```python
from build123d import *

# Parameters (mm, degrees)
SKETCH_1_R      = 5.05
SKETCH_1_R_2    = 2.05
SKETCH_1_R_3    = 3.701732688
EXTRUDE_1_DEPTH = 2


with BuildPart() as part:
    # 草图1 → 凸台-拉伸1 (new body)
    with BuildSketch(Plane.XY):
        with BuildLine():
            Line((-80.687991051, 42.414942906), (-80.687991051, -192.585057094))
            ThreePointArc((-80.687991051, -192.585057094), (-52.757273194, -260.015774951), (-120.187991051, -232.085057094))
            Line((-120.187991051, -232.085057094), (-140.687991051, -211.585057094))
            Line((-140.687991051, -211.585057094), (-140.687991051, 61.414942906))
            Line((-140.687991051, 61.414942906), (-120.187991051, 81.914942906))
            ThreePointArc((-120.187991051, 81.914942906), (-52.757273194, 109.845660763), (-80.687991051, 42.414942906))
        make_face()
        with Locations((-80.687991051, 81.914942906)):
            Circle(SKETCH_1_R, mode=Mode.SUBTRACT)
        with Locations((-80.687991051, 56.914942906)):
            Circle(SKETCH_1_R_2, mode=Mode.SUBTRACT)
        with Locations((-108.618708908, 53.984225049)):
            Circle(SKETCH_1_R_3, mode=Mode.SUBTRACT)
        with Locations((-55.687991051, 81.914942906)):
            Circle(SKETCH_1_R_2, mode=Mode.SUBTRACT)
        with Locations((-105.687991051, 81.914942906)):
            Circle(SKETCH_1_R_2, mode=Mode.SUBTRACT)
        with Locations((-80.687991051, 106.914942906)):
            Circle(SKETCH_1_R_2, mode=Mode.SUBTRACT)
        with Locations(Location((-80.687991051, -257.085057094, 0), (0, 0, 180))):
            Circle(SKETCH_1_R_2, mode=Mode.SUBTRACT)
        with Locations(Location((-105.687991051, -232.085057094, 0), (0, 0, 180))):
            Circle(SKETCH_1_R_2, mode=Mode.SUBTRACT)
        with Locations(Location((-55.687991051, -232.085057094, 0), (0, 0, 180))):
            Circle(SKETCH_1_R_2, mode=Mode.SUBTRACT)
        with Locations(Location((-108.618708908, -204.154339237, 0), (0, 0, 180))):
            Circle(SKETCH_1_R_3, mode=Mode.SUBTRACT)
        with Locations(Location((-80.687991051, -207.085057094, 0), (0, 0, 180))):
            Circle(SKETCH_1_R_2, mode=Mode.SUBTRACT)
        with Locations(Location((-80.687991051, -232.085057094, 0), (0, 0, 180))):
            Circle(SKETCH_1_R, mode=Mode.SUBTRACT)
    extrude(amount=EXTRUDE_1_DEPTH)


solid = part.part
```
Geometry: final body of the model. Coordinates: model frame, mm. Coordinates: 2 decimals unless noted, no trailing zeros. Order: outer loops, then holes, each group sorted by start corner. A loop starts at its lowest first (then second) coordinate and runs counter-clockwise, first axis right, second up. Notation, with made-up numbers: M 62,87 L 81,87 A27 ccw 81,103 Z; hole C 55.5,87 d11. An arc over 180 degrees is marked long. Answer in a Markdown table with one row per item. Add a question column.
Q1. Contact query for flat-ended pins moving along their axis: P1, Ø6.5, axis at x = -55.69, y = -232.09, coming from the +Z side; P2, Ø2.5, axis at x = -105.69, y = -232.09, coming from the +Z side; P3, Ø1, axis at y = -145.5, z = 0.5, coming from the +X side. Output: stop coordinate, or through.
Q2. Section query C-C on x = -98.5. Return the cut outline in (y, z).
Q3. Line query: L1, parallel to Y at x = -48.5, z = 0.6; L2, parallel to X at y = -21.5, z = 1.8; L3, parallel to Y at x = -55.5, z = 1.25. Output: solid intervals per line, ascending.
Q4. Section query B-B on y = -22. Return the cut outline in (x, z).
Q5. Section query A-A on z = 0.8. Count the separate pieces of the cut face and the enclosed holes in it, and give its area (3 significant figures).
Q6. Mould query, pull axis X, two halves, no side actions, for faces 1 (the flat face through (-130.294, -221.979, 0.986)), 2 (the cylindrical face through (-76.023, 79.981, 0.986)), 3 (the cylindrical face through (-53.69, 110.75, 0.99)). Classes: released by +X, released by -X, zero draft, split by the parting line, or undercut.
Completed:
| question | item | result |
|---|---|---|
| 1 | P1 | stops at z = 2 |
| 1 | P2 | passes through |
| 1 | P3 | stops at x = -80.69 |
| 2 | outline | M -267.34,0 L 117.17,0 L 117.17,2 L -267.34,2 Z |
| 3 | L1 | y = -254.98 to -209.19, 59.02 to 104.81 |
| 3 | L2 | x = -140.69 to -80.69 |
| 3 | L3 | y = -262.51 to -234.13, -230.04 to -201.66, 51.49 to 79.87, 83.96 to 112.34 |
| 4 | outline | M -140.69,0 L -80.69,0 L -80.69,2 L -140.69,2 Z |
| 5 | separate pieces | 1 |
| 5 | enclosed holes | 12 |
| 5 | area | 25,400 mm2 |
| 6 | face 1 | released by -X |
| 6 | face 2 | undercut |
| 6 | face 3 | split by the parting line |
